from build123d import *
from build123d.topology import SkipClean

# Parameters (mm, degrees)
BOSS_EXTRUDE1_DEPTH            = 17
CUT_EXTRUDE1_DEPTH             = 12
CUT_EXTRUDE2_DEPTH             = 35
CUT_EXTRUDE4_DEPTH             = 70
SKETCH8_R                      = 4
CUT_EXTRUDE5_DEPTH             = 47.01609876
CUT_EXTRUDE6_START             = -12.794651
SKETCH9_W                      = 3.3
SKETCH9_H                      = 13.87251724
CUT_EXTRUDE6_DEPTH             = 12.794651
F_2_5_2_5_DIAMETER_HOLE1_D     = 2.5
F_2_5_2_5_DIAMETER_HOLE1_DEPTH = 10
F_2_5_2_5_DIAMETER_HOLE1_TIP   = 0.751075774
SKETCH12_R                     = 2.25
SKETCH12_R_2                   = 1.25
EXTRUDE_THIN1_DEPTH            = 1.65
EXTRUDE_THIN1_TAPER            = -30
EXTRUDE_THIN1_OTHER_WAY_DEPTH  = 1.65
EXTRUDE_THIN1_OTHER_WAY_TAPER  = -30
SKETCH13_R                     = 1.25
CUT_EXTRUDE7_DEPTH             = 51.298409268
FILLET1_SIZE                   = 10
FILLET1_SIZE_2                 = 2


with BuildPart() as part:
    # Sketch1 → Boss-Extrude1 (new body)
    with BuildSketch(Plane.XY):
        Polygon((9.214105344, -17.845408642), (1.867831272, -10.231693567), (-6.924981548, 9.65081238), (-6.44974452, 27.27081238), (-2.341238634, 27.16), (-1.996273731, 39.95), (6.90049084, 39.710041319), (6.555525937, 26.920041319), (10.664031823, 26.80922894), (10.272676019, 12.29922894), (23.972676019, 10.97162784), (31.256458157, 3.422679717), (27.22651445, -0.465707315), (21.07453068, 5.910239336), (7.092065282, -7.581074959), (13.244049051, -13.95702161), align=None)
    extrude(amount=BOSS_EXTRUDE1_DEPTH)

    # Sketch3 → Cut-Extrude1 (cut)
    with BuildSketch(Plane(origin=(-3.071548911, 0.082844142, 0), x_dir=(0, 0, 1), z_dir=(-0.9996364686497187, 0.026961649532627044, 0))):
        with BuildLine():
            Line((0, 41.347002833), (0, 39.88165409))
            Line((0, 39.88165409), (11.85, 39.88165409))
            ThreePointArc((11.85, 39.88165409), (15.684994113, 36.06545508), (16.041740609, 30.667002833))
            Line((16.041740609, 30.667002833), (14.22, 27.087002833))
            Line((14.22, 27.087002833), (17.68, 27.087002833))
            Line((17.68, 27.087002833), (17.68, 41.347002833))
            Line((17.68, 41.347002833), (0, 41.347002833))
        make_face()
    extrude(amount=-CUT_EXTRUDE1_DEPTH, mode=Mode.SUBTRACT)

    # Sketch4 → Cut-Extrude2 (cut, symmetric)
    with BuildSketch(Plane(origin=(13.867127573, 13.38002785, 0), x_dir=(0, 0, 1), z_dir=(-0.7196328048525186, -0.6943548272894032, 0))):
        with BuildLine():
            Line((-2.314754212, -10.38), (0, -10.38))
            Line((0, -10.38), (0, -15.11))
            add(Edge.make_bspline(
                [(3.6, -17.452900819), (1.397081859, -16.752692527), (0, -15.11)],
                knots=[0, 0, 0, 1, 1, 1], degree=2))
            ThreePointArc((3.6, -17.452900819), (8.348973573, -18.829997515), (13.1, -17.46))
            Line((13.1, -17.46), (17, -17.46))
            Line((17, -17.46), (17, -10.38))
            Line((17, -10.38), (19.895245788, -10.38))
            Line((19.895245788, -10.38), (19.895245788, -23.53))
            Line((19.895245788, -23.53), (-2.314754212, -23.53))
            Line((-2.314754212, -23.53), (-2.314754212, -10.38))
        make_face()
    extrude(amount=CUT_EXTRUDE2_DEPTH, both=True, mode=Mode.SUBTRACT)

    # Sketch7 → Cut-Extrude4 (cut)
    with BuildSketch(Plane(origin=(-0.115337826, -0.111286444, 0), x_dir=(0, 0, -1), z_dir=(0.7196328048525139, 0.6943548272894081, 0))):
        with BuildLine():
            Line((-17, -17.46), (-13.094358857, -17.46))
            ThreePointArc((-13.094358857, -17.46), (-15.958832909, -14.422908382), (-17, -10.38))
            Line((-17, -10.38), (-17, -17.46))
        make_face()
    extrude(amount=-CUT_EXTRUDE4_DEPTH, mode=Mode.SUBTRACT)

    # Sketch8 → Cut-Extrude5 (cut, through all)
    with BuildSketch(Plane(origin=(17.89707128, 17.268414883, 0), x_dir=(0, 0, -1), z_dir=(0.7196328048525137, 0.6943548272894083, 0))):
        with Locations(Location((-8.5, -13.46, 0), (0, 0, 90))):
            Circle(SKETCH8_R)
    extrude(amount=-CUT_EXTRUDE5_DEPTH, mode=Mode.SUBTRACT)

    # Sketch9 → Cut-Extrude6 (cut)
    with SkipClean():  # the faces are left unmerged after this step: merging them gives an invalid solid
        with BuildSketch(Plane(origin=(1.07527518, 39.867155858, 0), x_dir=(0.9996364686497184, -0.026961649532630364, 0), z_dir=(0.026961649532630364, 0.9996364686497184, 0)).offset(CUT_EXTRUDE6_START)):
            with Locations((1.377334079, -9.43625862)):
                Rectangle(SKETCH9_W, SKETCH9_H)
        extrude(amount=CUT_EXTRUDE6_DEPTH, mode=Mode.SUBTRACT)

    # Ø2.5 (2.5) Diameter Hole1
    with Locations(Plane(origin=(-3.071548911, 0.082844142, 0), x_dir=(0, 0, 1), z_dir=(-0.9996364686497187, 0.026961649532627044, 0))):
        with Locations((8.8, 35.88165409)):
            Hole(F_2_5_2_5_DIAMETER_HOLE1_D / 2, depth=F_2_5_2_5_DIAMETER_HOLE1_DEPTH)
            with Locations((0, 0, -(F_2_5_2_5_DIAMETER_HOLE1_DEPTH + F_2_5_2_5_DIAMETER_HOLE1_TIP / 2))):  # 118° drill point
                Cone(0, F_2_5_2_5_DIAMETER_HOLE1_D / 2, F_2_5_2_5_DIAMETER_HOLE1_TIP, mode=Mode.SUBTRACT)

    # Sketch12 → Extrude-Thin1 (add)
    with SkipClean():  # the faces are left unmerged after this step: merging them gives an invalid solid
        with BuildSketch(Plane(origin=(1.376833375, -0.037135199, 0), x_dir=(0, 0, 1), z_dir=(-0.9996364686497184, 0.02696164953263036, 0))):
            with Locations((8.8, 35.88165409)):
                Circle(SKETCH12_R)
            with Locations((8.8, 35.88165409)):
                Circle(SKETCH12_R_2, mode=Mode.SUBTRACT)
        extrude(amount=-EXTRUDE_THIN1_DEPTH, taper=EXTRUDE_THIN1_TAPER)

    # Sketch12 → Extrude-Thin1 other way (add)
    with SkipClean():  # the faces are left unmerged after this step: merging them gives an invalid solid
        with BuildSketch(Plane(origin=(1.376833375, -0.037135199, 0), x_dir=(0, 0, 1), z_dir=(-0.9996364686497184, 0.02696164953263036, 0))):
            with Locations((8.8, 35.88165409)):
                Circle(SKETCH12_R)
            with Locations((8.8, 35.88165409)):
                Circle(SKETCH12_R_2, mode=Mode.SUBTRACT)
        extrude(amount=EXTRUDE_THIN1_OTHER_WAY_DEPTH, taper=EXTRUDE_THIN1_OTHER_WAY_TAPER)

    # Sketch13 → Cut-Extrude7 (cut, through all)
    with SkipClean():  # the faces are left unmerged after this step: merging them gives an invalid solid
        with BuildSketch(Plane(origin=(5.82521566, -0.157114539, 0), x_dir=(0, 0, -1), z_dir=(0.9996364686497184, -0.02696164953263123, 0))):
            with Locations(Location((-8.8, 35.88165409, 0), (0, 0, 270))):
                Circle(SKETCH13_R)
        extrude(amount=-CUT_EXTRUDE7_DEPTH, mode=Mode.SUBTRACT)

    # Fillet1
    # an asymmetric fillet: 10, 2 mm, written as the material it takes off along each edge
    with BuildSketch(Plane(origin=(-26.987185447, 40.624041238, 0), x_dir=(-0.02696164953263108, -0.9996364686497184, 0), z_dir=(0.9996364686497184, -0.02696164953263108, 0))) as fillet1_piece_1:
        with BuildLine():
            Bezier((FILLET1_SIZE, 0), (0, 0), (0, -FILLET1_SIZE_2), weights=[1, 0.707106781, 1])
            Line((0, -FILLET1_SIZE_2), (0, 0))
            Line((0, 0), (FILLET1_SIZE, 0))
        make_face()
    extrude(amount=58.9, mode=Mode.SUBTRACT)


solid = part.part
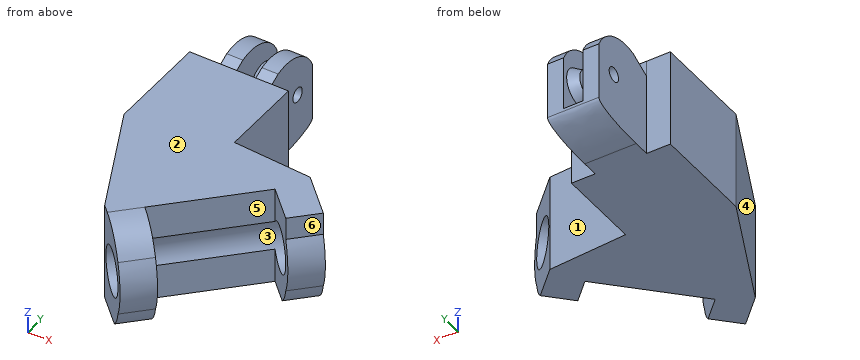
The model under review builds one solid part; all positions refer to its coordinate system, in mm. Face numbers are marked on the shaded views. A direction names the side the tool comes from. Coordinates: 2 decimals unless noted, no trailing zeros. Loops run counter-clockwise (first coordinate to the right, second up) from the corner with the lowest first, then second, coordinate; pieces in that order, holes last. Notation, with made-up numbers: (-18, 35.25) -> (-13, 35.25) arc R15 cw to (-13, 62.25) -> close; hole circle Ø2 at (53.5, 25.5). An arc over 180 degrees is marked (long way). Use a Markdown table: item, result. Add a question column.
1. Machinability: for the marked faces 5 and 6, which of the approach directions +Z, -Z, +X, -X, +Y, -Y give a long, thin tool a straight path to every point of the face, cutting with its end or side? Answer none if there is none.
2. Add section A-A on y = 21.5. Write out the cut boundary in (x, z), plus the area to 3 significant figures.
3. Clearance check with flat-ended pins moving along their axes: pin 1 Ø3 at (y, z) = (-7.5, 3) entering from -X; pin 2 Ø8 at (y, z) = (-4, 9) entering from +X; pin 3 Ø10 at (y, z) = (0.5, 15) entering from +X; pin 4 Ø2 at (x, y) = (22.5, 0.5) entering from -Z. State where each tip first meets the part, or that it passes through.
4. Draft analysis for pull direction X (two halves, no side actions). For the marked faces 1, 2, 3 and 4, state which applies: pulls with the +X half, pulls with the -X half, needs draft (parallel to the pull), parting line crosses it, or undercut.
5. To check wall thickness, follow line 1 (X direction, y = 2.5, z = 11); line 2 (Z direction, x = 5.5, y = -9); line 3 (X direction, y = 34, z = 4.75). State the ranges of each line that lie inside material, in increasing order.
Returned:
| question | item | result |
|---|---|---|
| 1 | face 5 | +Z, -Z |
| 1 | face 6 | +Z, +X, -Y |
| 2 | outline | (-6.61, 0) -> (10.52, 0) -> (10.52, 17) -> (-6.61, 17) -> close |
| 2 | area | 291 mm² |
| 3 | pin 1 | stops at x = 0 |
| 3 | pin 2 | stops at x = 27.1 |
| 3 | pin 3 | stops at x = 30.55 |
| 3 | pin 4 | passes through |
| 4 | face 1 | pulls with the +X half |
| 4 | face 2 | needs draft |
| 4 | face 3 | undercut |
| 4 | face 4 | pulls with the -X half |
| 5 | line 1 | x = -3.76 to 17.48, 26.47 to 29.13 |
| 5 | line 2 | z = 0 to 6.05, 10.95 to 17 |
| 5 | line 3 | x = -2.16 to 0.64, 3.95 to 6.75 |
